For this review, take the finished solid that the model builds, in its own axes (mm). Round coordinates to 2 decimals unless told otherwise and drop trailing zeros. Order: outer loops, then holes, each group sorted by start corner. A loop starts at its lowest first (then second) coordinate and runs counter-clockwise, first axis right, second up. Notation, with made-up numbers: M 81,11 L 138,11 A17 ccw 138,20 Z; hole C -9,-12.5 d8. An arc over 180 degrees is marked long. Put each result on its own line as item: value.
from build123d import *

# Parameters (mm, degrees)
F1_DEPTH = 914.4
F3_D     = 5.2197


with BuildPart() as f1:
    # F0 (on Right) → F1 (new body)
    with BuildSketch(Plane.YZ):
        with BuildLine():
            Line((0, 38.1), (0, 0))
            Line((0, 0), (1.27, 0))
            Line((1.27, 0), (1.27, 35.7240475594))
            ThreePointArc((1.27, 35.7240475594), (5.3775781238, 39.4470384182), (0, 38.1))
        make_face()
    extrude(amount=F1_DEPTH)

    # F3 (through all)
    with Locations(Plane.XZ):
        with Locations((38.1, 14.2875), (177.8, 14.2875), (317.5, 14.2875), (596.9, 14.2875), (736.6, 14.2875), (876.3, 14.2875), (457.2, 14.2875)):
            Hole(F3_D / 2)


solid = f1.part
(1) Add section B-B on x = 251. Give the boundary of the cut face in (y, z) (1 decimal), then the cut area to 3 significant figures.
A:
outline: M 0,0 L 1.3,0 L 1.3,35.7 A2.9 ccw long 0,38.1 Z
area: 71.9 mm2
(2) To check wall thickness, follow L1, parallel to Y at x = 63, z = 7; L2, parallel to Z at x = 254, y = 3.2; L3, parallel to Z at x = 826, y = 1.55. State the ranges of each line that lie inside material, in increasing order.
A:
L1: y = 0 to 1.27
L2: z = 35.26 to 40.94
L3: z = 35.56 to 40.64
(3) Insertion check: pin 1 Ø18 at (x, z) = (628, 18.5) entering from +Y. The pin has a flat end and moves straight along its axis. Give the tip position at first contact, or say it passes through.
A:
pin 1: stops at y = 1.27
(4) Add section A-A on z = 27. Give the boundary of the cut face in (x, y).
A:
outline: M 0,0 L 914.4,0 L 914.4,1.27 L 0,1.27 Z
